```python
from build123d import *

# Parameters (mm, degrees)
F0_W      = 38.1
F0_H      = 38.1
F1_DEPTH  = 38.1
F7_DEPTH  = 58.42
F8_DEPTH  = 38.1
F9_W      = 25.4
F9_H      = 7.62
F10_DEPTH = 63.5


with BuildPart() as f1:
    # F0 (on Front) → F1 (new body)
    with BuildSketch(Plane.XZ):
        Rectangle(F0_W, F0_H)
    extrude(amount=F1_DEPTH)

    # F5 (on offset) → F7 (cut)
    with BuildSketch(Plane.YZ.offset(38.1)):
        Polygon((-11.43, -5.783536), (-6.35, 19.05), (-31.75, 19.05), (-26.67, -3.85385), (-21.59, 9.525), (-16.51, 9.525), align=None)
        Polygon((-6.35, -19.05), (0, -19.05), (0, 19.05), align=None)
        Polygon((-25.4, -19.05), (-12.7, -19.05), (-19.05, -3.175), align=None)
        Polygon((-38.1, -19.05), (-31.75, -19.05), (-38.1, 19.05), align=None)
    extrude(amount=-F7_DEPTH, mode=Mode.SUBTRACT)

    # F6 (on offset) → F8 (cut)
    with BuildSketch(Plane.XZ.offset(38.1)):
        Polygon((6.35, 19.05), (-6.35, 19.05), (0, 3.175), align=None)
        Polygon((19.05, 19.05), (12.7, 19.05), (19.05, -19.05), align=None)
        Polygon((-7.62, 3.175), (-12.7, -19.05), (12.7, -19.05), (7.62, 3.175), (2.54, -9.507036), (-2.54, -9.507036), align=None)
        Polygon((-12.7, 19.05), (-19.05, 19.05), (-19.05, -19.05), align=None)
    extrude(amount=-F8_DEPTH, mode=Mode.SUBTRACT)

    # F9 (on offset) → F10 (cut)
    with BuildSketch(Plane.XY.offset(38.1)):
        with Locations((6.264115, -11.43)):
            Rectangle(F9_W, F9_H)
        with Locations((-6.435885, -26.67)):
            Rectangle(F9_W, F9_H)
    extrude(amount=-F10_DEPTH, mode=Mode.SUBTRACT)


solid = f1.part
```
Check sheet for the modelled part. Datum: model origin and axes. Units: mm. A direction names the side the tool comes from. Give positions to 0.01 mm unless a question says otherwise; leave off trailing zeros. Loops run counter-clockwise (first coordinate to the right, second up) from the corner with the lowest first, then second, coordinate; pieces in that order, holes last. Notation, with made-up numbers: M 29,77.5 L 83,77.5 A37 cw 83,116.5 Z; hole C 67.5,78 d2. An arc over 180 degrees is marked long. Answer in a Markdown table with one row per item.
1) Mould release check, pull along Y, two halves, no side actions. Record for faces 5 (the face through (8.065, -15.884, 7.638)), 6 (the face through (14.13, -22.18, -11)), 7 (the face through (9.63, -5.72, -5.62)): released by +Y, released by -Y, zero draft, split by the parting line, or undercut.
Solutions:
| item | result |
|---|---|
| face 5 | undercut |
| face 6 | undercut |
| face 7 | zero draft |
2) Depth check by flat-ended pin: pin 1 (12 mm diameter, centred on y = -12, z = 11.5, fed in from +X); pin 2 (0.6 mm diameter, centred on x = -0.5, y = -16, fed in from -Z); pin 3 (20.5 mm diameter, centred on x = 7, z = -10, fed in from -Y); pin 4 (1.5 mm diameter, centred on y = -28.5, z = 10, fed in from -X). Enter the tip coordinate at first touch or a pass-through.
Solutions:
| item | result |
|---|---|
| pin 1 | stops at x = 14.76 |
| pin 2 | stops at z = -9.51 |
| pin 3 | stops at y = -34.96 |
| pin 4 | passes through |
3) Cross-section at D-D (z = -14.5). Enter the section's corners in (x, y), plus the area to 3 significant figures.
Solutions:
| item | result |
|---|---|
| outline | M -18.29,-32.51 L -11.66,-32.51 L -11.66,-30.48 L -18.29,-30.48 Z; M -18.29,-14.52 L -11.66,-14.52 L -11.66,-5.59 L -18.29,-5.59 Z; M 11.66,-32.51 L 18.29,-32.51 L 18.29,-23.58 L 11.66,-23.58 Z; M 11.66,-7.62 L 18.29,-7.62 L 18.29,-5.59 L 11.66,-5.59 Z |
| area | 145 mm^2 |
4) Cross-section at A-A (y = -8.5). Enter the section's corners in (x, z) (3 decimals).
Solutions:
| item | result |
|---|---|
| outline | M -19.05,-19.05 L -12.7,-19.05 L -7.62,3.175 L -6.436,0.219 L -6.436,8.54 L -14.452,8.54 Z; M 18.964,-19.05 L 19.05,-19.05 L 18.964,-18.535 Z |
5) Thickness scan on line 1 (Y direction, x = 1.5, z = -1); line 2 (Y direction, x = 8, z = 8); line 3 (X direction, y = -7, z = -0.5). Record the ranges inside material, lowest first.
Solutions:
| item | result |
|---|---|
| line 1 | y = -34.76 to -30.48, -22.86 to -15.24, -7.62 to -3.34 |
| line 2 | y = -36.26 to -29.3, -22.17 to -16, -7.62 to -1.84 |
| line 3 | x = -15.96 to -8.46, -6.15 to 6.15, 8.46 to 15.96 |
6) Tool access check on faces 1 (the face through (0.07, -18.05, -5.68)), 2 (the face through (5.6, -15.24, -1.3)), 3 (the face through (-3.22, -33.5, 11.22)), 4 (the face through (0, -22, -9.507)). Record the directions out of +Z, -Z, +X, -X, +Y, -Y that give a thin tool (end or side, any length) a straight path to the whole face; none if there is none.
Solutions:
| item | result |
|---|---|
| face 1 | -Z, +X, -X |
| face 2 | +Z, -Z, +X |
| face 3 | +Z, +Y, -Y |
| face 4 | -Z, +Y, -Y |
7) Cross-section at C-C (z = 7). Enter the section's corners in (x, y).
Solutions:
| item | result |
|---|---|
| outline | M -14.71,-36.09 L -1.53,-36.09 L -1.53,-30.48 L -14.71,-30.48 Z; M -14.71,-22.55 L -1.53,-22.55 L -1.53,-15.67 L -14.71,-15.67 Z; M -14.71,-8.81 L -6.44,-8.81 L -6.44,-7.62 L -1.53,-7.62 L -1.53,-2.01 L -14.71,-2.01 Z; M 1.53,-36.09 L 14.71,-36.09 L 14.71,-29.08 L 6.26,-29.08 L 6.26,-30.48 L 1.53,-30.48 Z; M 1.53,-22.55 L 14.71,-22.55 L 14.71,-15.67 L 1.53,-15.67 Z; M 1.53,-7.62 L 14.71,-7.62 L 14.71,-2.01 L 1.53,-2.01 Z |
